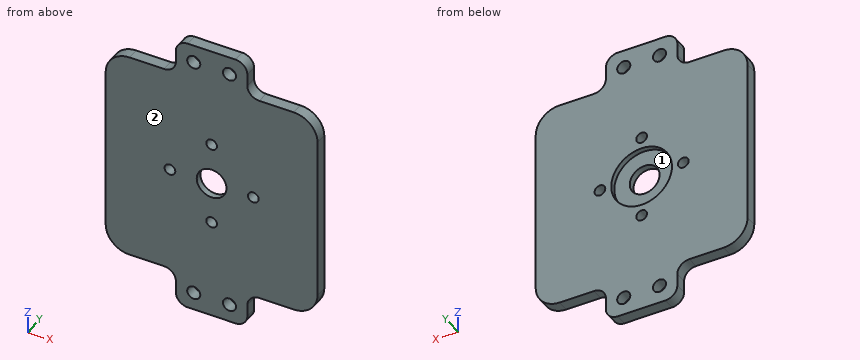
from build123d import *

# Parameters (mm, degrees)
SKETCH1_R           = 2.25
SKETCH1_R_2         = 2.75
SKETCH1_R_3         = 6.25
BOSS_EXTRUDE1_DEPTH = 5
FILLET1_R           = 10
FILLET2_R           = 5
SKETCH2_R           = 12.75
CUT_EXTRUDE1_DEPTH  = 2.25


with BuildPart() as part:
    # Sketch1 → Boss-Extrude1 (new body)
    with BuildSketch(Plane(origin=(0, 0, 0), x_dir=(1, 0, 0), z_dir=(0, 1, 0))):
        Polygon((0, 88.9), (0, 0), (29.45, 0), (29.45, -15), (59.45, -15), (59.45, 0), (88.9, 0), (88.9, 88.9), (59.45, 88.9), (59.45, 103.9), (29.45, 103.9), (29.45, 88.9), align=None)
        with Locations(Location((61.95, 44.45, 0), (0, 0, 270))):
            Circle(SKETCH1_R, mode=Mode.SUBTRACT)
        with Locations(Location((44.45, 26.95, 0), (0, 0, 270))):
            Circle(SKETCH1_R, mode=Mode.SUBTRACT)
        with Locations(Location((26.95, 44.45, 0), (0, 0, 270))):
            Circle(SKETCH1_R, mode=Mode.SUBTRACT)
        with Locations(Location((44.45, 61.95, 0), (0, 0, 270))):
            Circle(SKETCH1_R, mode=Mode.SUBTRACT)
        with Locations(Location((36.95, -7.5, 0), (0, 0, 270))):
            Circle(SKETCH1_R_2, mode=Mode.SUBTRACT)
        with Locations(Location((51.95, -7.5, 0), (0, 0, 270))):
            Circle(SKETCH1_R_2, mode=Mode.SUBTRACT)
        with Locations(Location((36.95, 96.4, 0), (0, 0, 270))):
            Circle(SKETCH1_R_2, mode=Mode.SUBTRACT)
        with Locations(Location((51.95, 96.4, 0), (0, 0, 270))):
            Circle(SKETCH1_R_2, mode=Mode.SUBTRACT)
        with Locations(Location((44.45, 44.45, 0), (0, 0, 270))):
            Circle(SKETCH1_R_3, mode=Mode.SUBTRACT)
    extrude(amount=BOSS_EXTRUDE1_DEPTH)

    # Fillet1
    fillet1_edges = [part.edges().sort_by_distance(p)[0] for p in [
        (0, 2.5, 0),
        (0, 2.5, -88.9),
        (88.9, 2.5, -88.9),
        (88.9, 2.5, 0),
    ]]
    fillet(fillet1_edges, radius=FILLET1_R)

    # Fillet2
    fillet2_edges = [part.edges().sort_by_distance(p)[0] for p in [
        (29.45, 2.5, 15),
        (29.45, 2.5, 0),
        (29.45, 2.5, -88.9),
        (29.45, 2.5, -103.9),
        (59.45, 2.5, -103.9),
        (59.45, 2.5, -88.9),
        (59.45, 2.5, 0),
        (59.45, 2.5, 15),
    ]]
    fillet(fillet2_edges, radius=FILLET2_R)

    # Sketch2 → Cut-Extrude1 (cut)
    with BuildSketch(Plane(origin=(0, 5, 0), x_dir=(1, 0, 0), z_dir=(0, 1, 0))):
        with Locations(Location((44.45, 44.45, 0), (0, 0, 270))):
            Circle(SKETCH2_R)
    extrude(amount=-CUT_EXTRUDE1_DEPTH, mode=Mode.SUBTRACT)


solid = part.part
Here's how the part is built. I have some questions about the finished solid (model axes, mm). Face numbers are marked on the shaded views. Coordinates: 2 decimals unless noted, no trailing zeros. Order: outer loops, then holes, each group sorted by start corner. A loop starts at its lowest first (then second) coordinate and runs counter-clockwise, first axis right, second up. Notation, with made-up numbers: M 55,60 L 75,60 A28 cw 75,84 Z; hole C -37.75,-19.5 d5. An arc over 180 degrees is marked long. Answer as CSV lines item,"result".
Item 1: Imagine slicing it at A-A on z = 7.5. Write out the boundary of the cut face in (x, y).
Results found:
outline,"M 29.45,0 L 34.2,0 L 34.2,5 L 29.45,5 Z; M 39.7,0 L 49.2,0 L 49.2,5 L 39.7,5 Z; M 54.7,0 L 59.45,0 L 59.45,5 L 54.7,5 Z"
Item 2: Imagine slicing it at D-D on z = -26.95. Write out the boundary of the cut face in (x, y), plus the area to 3 significant figures.
Results found:
outline,"M 0,0 L 42.2,0 L 42.2,5 L 0,5 Z; M 46.7,0 L 88.9,0 L 88.9,5 L 46.7,5 Z"
area,"422 mm2"
Item 3: For pin 1 (2.5 mm diameter, centred on y = 2.5, z = -97, fed in from -X); pin 2 (14.5 mm diameter, centred on x = 44.45, z = -44.45, fed in from +Y); pin 3 (1.5 mm diameter, centred on x = 69, y = 1.5, fed in from -Z), each with a flat end and sliding along its axis, tell me the tip position at first contact or that it passes through.
Results found:
pin 1,"x = 29.45"
pin 2,"y = 2.75"
pin 3,"z = -88.9"
Item 4: We'd pull the mould along Z, two halves only. Please class the marked faces 1 and 2: +Z half, -Z half, draft (parallel to the pull), parting line (faces both ways), or undercut.
Results found:
face 1,"undercut"
face 2,"draft"
Item 5: Imagine slicing it at C-C on y = 3.8. Give the number of separate pieces and of enclosed holes in the cut face, plus the area to 3 significant figures.
Results found:
separate pieces,"1"
enclosed holes,"9"
area,"8,050 mm2"
Item 6: Imagine slicing it at B-B on x = 44.45. Write out the boundary of the cut face in (y, z).
Results found:
outline,"M 0,-103.9 L 5,-103.9 L 5,-64.2 L 0,-64.2 Z; M 0,-59.7 L 5,-59.7 L 5,-57.2 L 2.75,-57.2 L 2.75,-50.7 L 0,-50.7 Z; M 0,-38.2 L 2.75,-38.2 L 2.75,-31.7 L 5,-31.7 L 5,-29.2 L 0,-29.2 Z; M 0,-24.7 L 5,-24.7 L 5,15 L 0,15 Z"
Item 7: If I drill on line 1 (X direction, y = 3.2, z = -44.5); line 2 (X direction, y = 2.6, z = -44.45); line 3 (X direction, y = 3.45, z = -96.4), over which ranges is the centre line in solid material (lowest first)?
Results found:
line 1,"0 to 24.7, 29.2 to 31.7, 57.2 to 59.7, 64.2 to 88.9"
line 2,"0 to 24.7, 29.2 to 38.2, 50.7 to 59.7, 64.2 to 88.9"
line 3,"29.45 to 34.2, 39.7 to 49.2, 54.7 to 59.45"
